Input: part model. Units: mm. Frame: model coordinates. A direction names the side the tool comes from. Coordinates: 2 decimals unless noted, no trailing zeros. Order: outer loops, then holes, each group sorted by start corner. A loop starts at its lowest first (then second) coordinate and runs counter-clockwise, first axis right, second up. Notation, with made-up numbers: (80, 17.5) - (85, 17.5) arc R14 cw to (85, 30.5) - close; hole circle Ø3 at (12.25, 13.5). An arc over 180 degrees is marked (long way). Use a Markdown table: item, result. Add a question column.
from build123d import *

# Parameters (mm, degrees)
SKETCH_1_W           = 41
SKETCH_1_H           = 23
EXTRUDE_1_DEPTH      = 13
EXTRUDE_2_DEPTH      = 15
EXTRUDE_2_DEPTH_BACK = 21
SKETCH_2_R           = 2.5
EXTRUDE_3_DEPTH      = 2
EXTRUDE_3_DEPTH_BACK = 22
SKETCH_3_R           = 2
SKETCH_3_R_2         = 2.5
CUT_EXTRUDE_1_DEPTH  = 7
CUT_EXTRUDE_2_DEPTH  = 8
EXTRUDE_4_DEPTH      = 15
EXTRUDE_5_DEPTH      = 16
EXTRUDE_10_DEPTH     = 9
EXTRUDE_7_DEPTH      = 1
SKETCH_12_W          = 1
SKETCH_12_H          = 4.898979486
EXTRUDE_11_DEPTH     = 21.5
SKETCH_13_W          = 19
SKETCH_13_H          = 4.898979486
EXTRUDE_12_DEPTH     = 1


with BuildPart() as part:
    # 스케치1 → 보스-돌출1 (new body)
    with BuildSketch(Plane(origin=(0, 0, 0), x_dir=(0, 0, -1), z_dir=(1, 0, 0))):
        Rectangle(SKETCH_1_W, SKETCH_1_H)
    extrude(amount=-EXTRUDE_1_DEPTH)

    # 스케치2 → 보스-돌출2 (add, two sides: drawn at the far end of the back side and taken through both)
    with BuildSketch(Plane(origin=(0, 0, 0), x_dir=(0, 0, -1), z_dir=(1, 0, 0)).offset(-EXTRUDE_2_DEPTH_BACK)):
        with Locations((-9.5, 0)):
            Circle(SKETCH_2_R)
    extrude(amount=EXTRUDE_2_DEPTH + EXTRUDE_2_DEPTH_BACK)

    # 스케치3 → 보스-돌출3 (add, two sides: drawn at the far end of the back side and taken through both)
    with BuildSketch(Plane.ZY.offset(13).offset(-EXTRUDE_3_DEPTH_BACK)):
        with Locations((-2, 0)):
            Circle(SKETCH_3_R)
        with Locations(Location((9.5, 0, 0), (0, 0, 180))):
            Circle(SKETCH_3_R_2)
    extrude(amount=EXTRUDE_3_DEPTH + EXTRUDE_3_DEPTH_BACK)

    # 스케치5 → 컷-돌출1 (cut)
    with BuildSketch(Plane.ZY.offset(21)):
        with BuildLine():
            Line((7.5, 1.5), (11.5, 1.5))
            ThreePointArc((11.5, 1.5), (9.5, 2.5), (7.5, 1.5))
        make_face()
        with BuildLine():
            Line((7.5, -1.5), (11.5, -1.5))
            ThreePointArc((11.5, -1.5), (9.5, -2.5), (7.5, -1.5))
        make_face()
    extrude(amount=-CUT_EXTRUDE_1_DEPTH, mode=Mode.SUBTRACT)

    # 스케치6 → 컷-돌출2 (cut)
    with BuildSketch(Plane(origin=(15, 0, 0), x_dir=(0, 0, -1), z_dir=(1, 0, 0))):
        with BuildLine():
            Line((-11.5, 1.5), (-7.5, 1.5))
            ThreePointArc((-7.5, 1.5), (-9.5, 2.5), (-11.5, 1.5))
        make_face()
        with BuildLine():
            Line((-11.5, -1.5), (-7.5, -1.5))
            ThreePointArc((-7.5, -1.5), (-9.5, -2.5), (-11.5, -1.5))
        make_face()
    extrude(amount=-CUT_EXTRUDE_2_DEPTH, mode=Mode.SUBTRACT)

    # 스케치7 → 보스-돌출4 (add)
    with BuildSketch(Plane(origin=(0, 0, 0), x_dir=(0, 0, -1), z_dir=(1, 0, 0))):
        with BuildLine():
            Line((3.5, 7.5), (3.5, -7.5))
            ThreePointArc((3.5, -7.5), (12, -11.5), (20.5, -7.5))
            Line((20.5, -7.5), (20.5, 7.5))
            ThreePointArc((20.5, 7.5), (12, 11.5), (3.5, 7.5))
        make_face()
    extrude(amount=EXTRUDE_4_DEPTH)

    # 스케치8 → 보스-돌출5 (add)
    with BuildSketch(Plane(origin=(15, 0, 0), x_dir=(0, 0, -1), z_dir=(1, 0, 0))):
        with BuildLine():
            Line((4.5, 7.130279596), (4.5, -7.130279596))
            ThreePointArc((4.5, -7.130279596), (12, -10.5), (19.5, -7.130279596))
            Line((19.5, -7.130279596), (19.5, 7.130279596))
            ThreePointArc((19.5, 7.130279596), (12, 10.5), (4.5, 7.130279596))
        make_face()
    extrude(amount=EXTRUDE_5_DEPTH)

    # 스케치10 → 보스-돌출10 (add)
    with BuildSketch(Plane(origin=(0, 0, 0), x_dir=(0, 0, -1), z_dir=(1, 0, 0))):
        with BuildLine():
            ThreePointArc((20.5, 1.322875656), (20, 0), (20.5, -1.322875656))
            Line((20.5, -1.322875656), (20.5, 1.322875656))
        make_face()
        with BuildLine():
            Line((20.5, 1.322875656), (20.5, -1.322875656))
            ThreePointArc((20.5, -1.322875656), (21.177124344, -1.822875656), (22, -2))
            ThreePointArc((22, -2), (23.414213562, -1.414213562), (24, 0))
            ThreePointArc((24, 0), (23.414213562, 1.414213562), (22, 2))
            ThreePointArc((22, 2), (21.177124344, 1.822875656), (20.5, 1.322875656))
        make_face()
    extrude(amount=EXTRUDE_10_DEPTH)

    # 스케치11 → 보스-돌출7 (add)
    with BuildSketch(Plane(origin=(9, 0, 0), x_dir=(0, 0, -1), z_dir=(1, 0, 0))):
        with BuildLine():
            Line((20, -1.5), (20, 1.5))
            ThreePointArc((20, 1.5), (24.5, 0), (20, -1.5))
        make_face()
        with BuildLine():
            Line((4, -1.5), (4, 1.5))
            ThreePointArc((4, 1.5), (-0.5, 0), (4, -1.5))
        make_face()
    extrude(amount=EXTRUDE_7_DEPTH)

    # 스케치12 → 보스-돌출11 (add)
    with BuildSketch(Plane(origin=(10, 0, 0), x_dir=(0, 0, -1), z_dir=(1, 0, 0))):
        with Locations((21, 0)):
            Rectangle(SKETCH_12_W, SKETCH_12_H)
        with Locations((3, 0)):
            Rectangle(SKETCH_12_W, SKETCH_12_H)
    extrude(amount=EXTRUDE_11_DEPTH)

    # 스케치13 → 보스-돌출12 (add)
    with BuildSketch(Plane(origin=(31.5, 0, 0), x_dir=(0, 0, -1), z_dir=(1, 0, 0))):
        with Locations((12, 0)):
            Rectangle(SKETCH_13_W, SKETCH_13_H)
    extrude(amount=EXTRUDE_12_DEPTH)


solid = part.part
1) Cut plane A-A (x = 19). Return the cut outline in (y, z), and give its area (3 significant figures).
2) Contact query for flat-ended pins moving along their axis: P1, Ø2, axis at x = 12.5, y = 2, coming from the -Z side; P2, Ø1.9, axis at x = 5, y = -4, coming from the +Z side; P3, Ø10, axis at y = 6, z = 15.5, coming from the +X side. Output: stop coordinate, or through.
3) Reachability of faces 5 (the flat face through (23, 0, -4.5)), 6 (the flat face through (11, -1.5, 10)), 7 (the cylindrical face through (5.728, 0.751, 7.115)), 8 (the cylindrical face through (-14, -2, -2)), 9 (the flat face through (-15, 0, -2)) from +Z, -Z, +X, -X, +Y, -Y: full face, straight path, thin tool, end or side. Return the list, or none.
4) Pull-direction query (X, two-part tool) for faces 1 (the flat face through (10, 0, -1)), 2 (the cylindrical face through (5, 0, 0)), 3 (the cylindrical face through (7.4, 11.5, -12.1)), 4 (the flat face through (31.5, 0, -12)); classes: pulls with the +X half, pulls with the -X half, needs draft (parallel to the pull), parting line crosses it, or undercut.
5) Material intervals for L1, parallel to Z at x = 26.5, y = -1; L2, parallel to Z at x = 16, y = -6.5; L3, parallel to X at y = -3.25, z = 6, sorted ascending.
6) Cut plane B-B (x = 4). Return the cut outline in (y, z).
7) Cut plane D-D (y = 4). Return the cut outline in (x, z).
8) Cut plane C-C (z = -18.5). Return the cut outline in (x, y), and give its area (3 significant figures).
Computed:
| question | item | result |
|---|---|---|
| 1 | outline | (-7.13, -19.5) - (7.13, -19.5) arc R10.03 ccw to (7.13, -4.5) - (-7.13, -4.5) arc R10.03 ccw to start; (-2.45, -21.5) - (2.45, -21.5) - (2.45, -20.5) - (-2.45, -20.5) - close; (-2.45, -3.5) - (2.45, -3.5) - (2.45, -2.5) - (-2.45, -2.5) - close |
| 1 | area | 294 mm2 |
| 2 | P1 | stops at z = -21.5 |
| 2 | P2 | stops at z = -3.5 |
| 2 | P3 | stops at x = 0 |
| 3 | face 5 | +Y, -Y |
| 3 | face 6 | +Z, +X, -Y |
| 3 | face 7 | +X |
| 3 | face 8 | -X |
| 3 | face 9 | -Z, -X, +Y, -Y |
| 4 | face 1 | pulls with the +X half |
| 4 | face 2 | undercut |
| 4 | face 3 | needs draft |
| 4 | face 4 | undercut |
| 5 | L1 | z = -21.5 to -20.5, -19.5 to -4.5, -3.5 to -2.5 |
| 5 | L2 | z = -19.5 to -4.5 |
| 5 | L3 | x = -13 to 0 |
| 6 | outline | (-7.5, -20.5) - (-1.32, -20.5) arc R2 ccw (long way) to (1.32, -20.5) - (7.5, -20.5) arc R11.03 ccw to (7.5, -3.5) - (1.32, -3.5) arc R2 ccw (long way) to (-1.32, -3.5) - (-7.5, -3.5) arc R11.03 ccw to start; circle Ø5 at (0, 9.5) |
| 7 | outline | (-13, -20.5) - (15, -20.5) - (15, -19.5) - (31, -19.5) - (31, -4.5) - (15, -4.5) - (15, -3.5) - (0, -3.5) - (0, 20.5) - (-13, 20.5) - close |
| 8 | outline | (-13, -11.5) - (0, -11.5) - (0, -9.38) - (15, -9.38) - (15, -8.11) - (31, -8.11) - (31, 8.11) - (15, 8.11) - (15, 9.38) - (0, 9.38) - (0, 11.5) - (-13, 11.5) - close; (31.5, -2.45) - (32.5, -2.45) - (32.5, 2.45) - (31.5, 2.45) - close |
| 8 | area | 845 mm2 |
